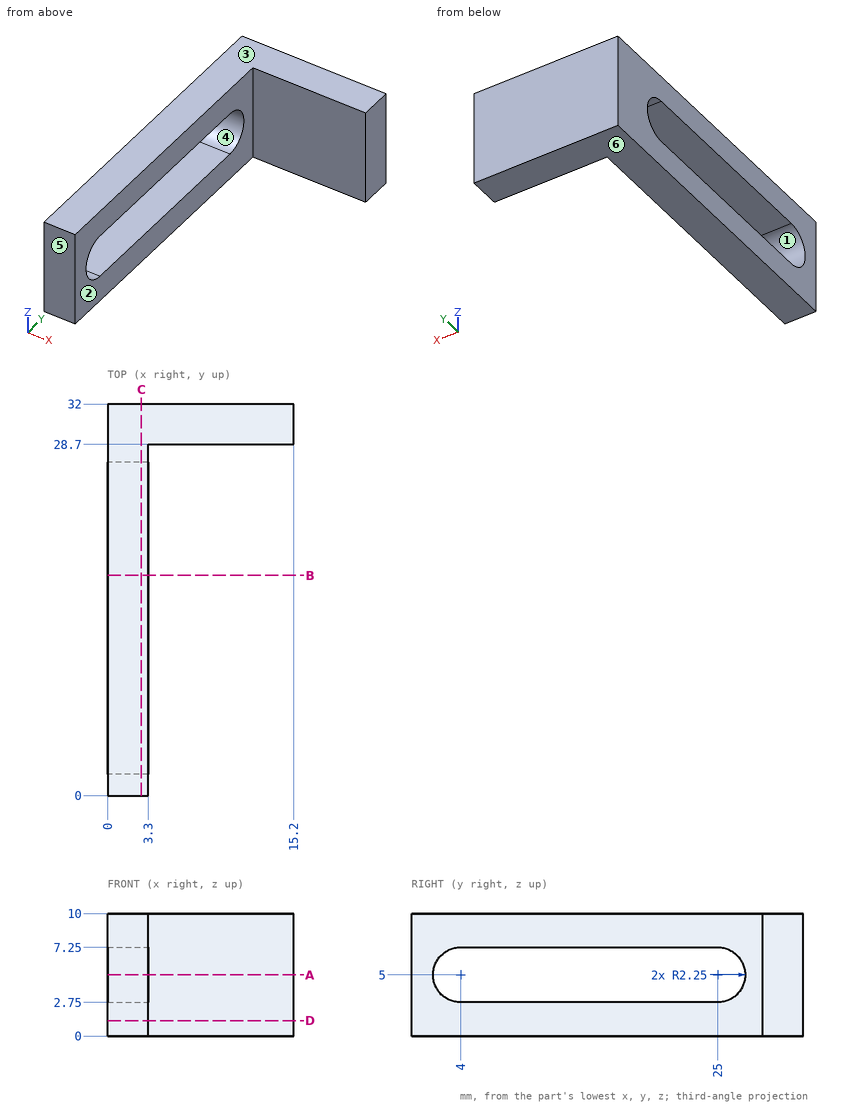
Part print with two shaded views. Sizes in mm from the minimum x, y, z corner. A direction names the side the tool comes from. Give positions to 0.01 mm unless a question says otherwise; leave off trailing zeros. Order: outer loops, then holes, each group sorted by start corner. A loop starts at its lowest first (then second) coordinate and runs counter-clockwise, first axis right, second up.
1) Saw through at C-C, the plane x = 2.75. Write the cut outline in (y, z), then the cut area to 3 significant figures.
2) Saw through at B-B, the plane y = 18. Write the cut outline in (x, z), then the cut area to 4 significant figures.
3) Mould opens along Z. For the marked faces 4, 5 and 6 say: +Z half, -Z half, draft (parallel to the pull), parting line (faces both ways), or undercut.
4) Saw through at D-D, the plane z = 1.25. Write the cut outline in (x, y).
5) Wall check: probe 1 along Z at (x, y) = (3.25, 18); probe 2 along Y at (x, z) = (9.5, 8.75); probe 3 along X at (y, z) = (11.5, 7.5). Give the ranges that are in metal, low to high.
6) Saw through at A-A, the plane z = 5. Write the cut outline in (x, y), then the cut area to 3 significant figures.
7) Pin check, flat tips, straight feed: pin 1 (3 mm diameter, centred on x = 11, z = 7.5, fed in from -Y); pin 2 (4 mm diameter, centred on y = 6.5, z = 3.5, fed in from +X). Stop position of each tip, or through.
8) 3-axis set-ups, long thin cutter, end or side, ignore diameter. For the marked faces 1, 2 and 3: which of +Z, -Z, +X, -X, +Y, -Y reach the whole face in a straight line?
Computed:
1. outline: (0, 0) - (32, 0) - (32, 10) - (0, 10) - close; hole (4, 2.75) - (25, 2.75) arc R2.25 ccw to (25, 7.25) - (4, 7.25) arc R2.25 ccw to start
1. area: 210 mm2
2. outline: (0, 0) - (3.3, 0) - (3.3, 2.75) - (0, 2.75) - close; (0, 7.25) - (3.3, 7.25) - (3.3, 10) - (0, 10) - close
2. area: 18.15 mm2
3. face 4: undercut
3. face 5: draft
3. face 6: -Z half
4. outline: (0, 0) - (3.3, 0) - (3.3, 28.7) - (15.2, 28.7) - (15.2, 32) - (0, 32) - close
5. probe 1: z = 0 to 2.75, 7.25 to 10
5. probe 2: y = 28.7 to 32
5. probe 3: x = 0 to 3.3
6. outline: (0, 0) - (3.3, 0) - (3.3, 1.75) - (0, 1.75) - close; (0, 27.25) - (3.3, 27.25) - (3.3, 28.7) - (15.2, 28.7) - (15.2, 32) - (0, 32) - close
6. area: 60.7 mm2
7. pin 1: stops at y = 28.7
7. pin 2: stops at x = 3.3
8. face 1: +X, -X
8. face 2: +Z, -Z, +X, -Y
8. face 3: +Z, +X, -X, +Y, -Y
